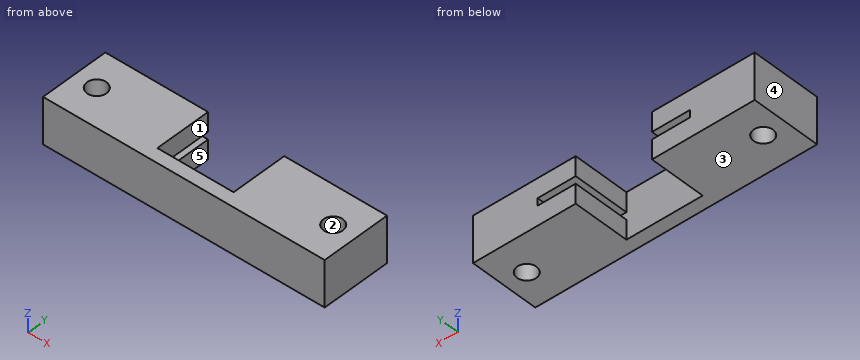
from build123d import *

# Parameters (mm, degrees)
BOSS_EXTRUDE1_DEPTH   = 8.7
BOSS_EXTRUDE1_2_DEPTH = 8.7
SKETCH3_W             = 29.6
SKETCH3_H             = 7.13
BOSS_EXTRUDE2_DEPTH   = 2
SKETCH4_W             = 7
SKETCH4_H             = 10.7
SKETCH4_R             = 1.5
BOSS_EXTRUDE3_DEPTH   = 7.13


with BuildPart() as part:
    # Sketch2 → Boss-Extrude1 (new body)
    with BuildSketch(Plane(origin=(0, 0, 0), x_dir=(1, 0, 0), z_dir=(0, 1, 0))):
        Polygon((-5.9, 3.565), (-5.9, 0.565), (-11.8, 0.565), (-11.8, -0.565), (-5.9, -0.565), (-5.9, -3.565), (-14.8, -3.565), (-14.8, 3.565), align=None)
    extrude(amount=BOSS_EXTRUDE1_DEPTH)



with BuildPart() as body_2:
    # Sketch2 → Boss-Extrude1 2 (new body)
    with BuildSketch(Plane(origin=(0, 0, 0), x_dir=(1, 0, 0), z_dir=(0, 1, 0))):
        Polygon((5.9, -0.565), (11.8, -0.565), (11.8, 0.565), (5.9, 0.565), (5.9, 3.565), (14.8, 3.565), (14.8, -3.565), (5.9, -3.565), align=None)
    extrude(amount=BOSS_EXTRUDE1_2_DEPTH)


with BuildPart() as part_1:
    add(part.part)

    add(body_2.part)  # Boss-Extrude2 merges body 2
    # Sketch3 → Boss-Extrude2 (add)
    with BuildSketch(Plane.XZ):
        Rectangle(SKETCH3_W, SKETCH3_H)
    extrude(amount=BOSS_EXTRUDE2_DEPTH)

    # Sketch4 → Boss-Extrude3 (add)
    with BuildSketch(Plane.XY.offset(3.565)):
        with Locations((18.3, 3.35)):
            Rectangle(SKETCH4_W, SKETCH4_H)
        with Locations((18.3, 3.35)):
            Circle(SKETCH4_R, mode=Mode.SUBTRACT)
        with Locations((-18.3, 3.35)):
            Rectangle(SKETCH4_W, SKETCH4_H)
        with Locations((-18.3, 3.35)):
            Circle(SKETCH4_R, mode=Mode.SUBTRACT)
    extrude(amount=-BOSS_EXTRUDE3_DEPTH)


solid = part_1.part
Can you work these out from the model? Positions are in its coordinate system, mm. Face numbers are marked on the shaded views. A direction names the side the tool comes from. Give positions to 0.01 mm unless a question says otherwise; leave off trailing zeros. Write each loop counter-clockwise with the first axis right and the second up, starting at its lowest first coordinate (ties: lowest second). Pieces come first, ordered by that corner, then holes. Notation, with made-up numbers: M -20,-6.75 L 35,-6.75 A23 ccw 35,17.25 Z; hole C 25.5,66 d7. An arc over 180 degrees is marked long. Answer in a Markdown table with one row per item. Add a question column.
Item 1: Imagine slicing it at D-D, the plane y = 3.35. Write out the boundary of the cut face in (x, z) (3 decimals).
Item 2: We'd pull the mould along X, two halves only. Please class the marked faces 3, 4 and 5: released by +X, released by -X, zero draft, split by the parting line, or undercut.
Item 3: On a 3-axis mill with a long thin cutter (end or side, diameter ignored), from which of +Z, -Z, +X, -X, +Y, -Y can I reach the whole of each face in a straight line? I mean the marked faces 1 and 2. Say none if no direction works.
Item 4: Please list where these lines run through material, in increasing order: L1, parallel to X at y = 7.25, z = -0.75; L2, parallel to Z at x = 10.5, y = 1.25 (3 decimals); L3, parallel to Y at x = -18.3, z = -1.25.
Item 5: Imagine slicing it at C-C, the plane x = 18.3. Write out the boundary of the cut face in (y, z) (3 decimals), plus the area to 3 significant figures.
Item 6: Imagine slicing it at A-A, the plane y = 6. Write out the boundary of the cut face in (x, z) (3 decimals).
Item 7: For pin 1 Ø1 at (x, z) = (4, 2.5) entering from +Y, with a flat end and sliding along its axis, tell me the tip position at first contact or that it passes through.
Item 8: Imagine slicing it at B-B, the plane z = -1.5. Write out the boundary of the cut face in (x, y).
Evaluation:
| question | item | result |
|---|---|---|
| 1 | outline | M -21.8,-3.565 L -19.8,-3.565 L -19.8,3.565 L -21.8,3.565 Z; M -16.8,-3.565 L -5.9,-3.565 L -5.9,-0.565 L -11.8,-0.565 L -11.8,0.565 L -5.9,0.565 L -5.9,3.565 L -16.8,3.565 Z; M 5.9,-3.565 L 16.8,-3.565 L 16.8,3.565 L 5.9,3.565 L 5.9,0.565 L 11.8,0.565 L 11.8,-0.565 L 5.9,-0.565 Z; M 19.8,-3.565 L 21.8,-3.565 L 21.8,3.565 L 19.8,3.565 Z |
| 2 | face 3 | zero draft |
| 2 | face 4 | released by -X |
| 2 | face 5 | undercut |
| 3 | face 1 | +Z, -Z, +Y |
| 3 | face 2 | +Z, -Z |
| 4 | L1 | x = -21.8 to -5.9, 5.9 to 21.8 |
| 4 | L2 | z = -3.565 to -0.565, 0.565 to 3.565 |
| 4 | L3 | y = -2 to 1.85, 4.85 to 8.7 |
| 5 | outline | M -2,-3.565 L 1.85,-3.565 L 1.85,3.565 L -2,3.565 Z; M 4.85,-3.565 L 8.7,-3.565 L 8.7,3.565 L 4.85,3.565 Z |
| 5 | area | 54.9 mm² |
| 6 | outline | M -21.8,-3.565 L -5.9,-3.565 L -5.9,-0.565 L -11.8,-0.565 L -11.8,0.565 L -5.9,0.565 L -5.9,3.565 L -21.8,3.565 Z; M 5.9,-3.565 L 21.8,-3.565 L 21.8,3.565 L 5.9,3.565 L 5.9,0.565 L 11.8,0.565 L 11.8,-0.565 L 5.9,-0.565 Z |
| 7 | pin 1 | stops at y = 0 |
| 8 | outline | M -21.8,-2 L 21.8,-2 L 21.8,8.7 L 5.9,8.7 L 5.9,0 L -5.9,0 L -5.9,8.7 L -21.8,8.7 Z; hole C -18.3,3.35 d3; hole C 18.3,3.35 d3 |
